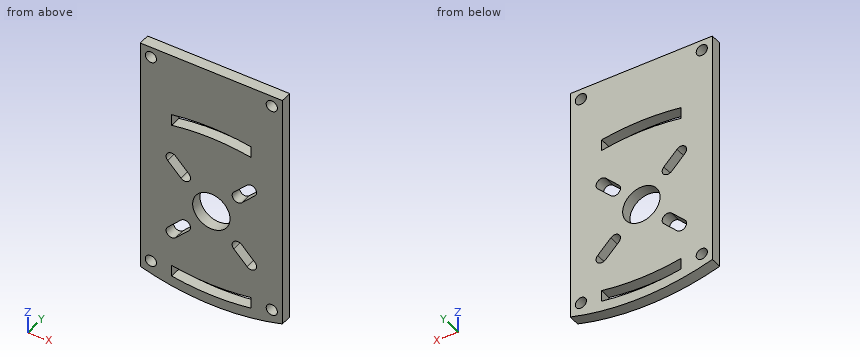
```python
from build123d import *

# Parameters (mm, degrees)
SKETCH_1_R      = 5
SKETCH_1_R_2    = 1.5
EXTRUDE_2_DEPTH = 3


with BuildPart() as part:
    # 草图1 → 凸台-拉伸2 (new body)
    with BuildSketch(Plane(origin=(0, 0, 0), x_dir=(1, 0, 0), z_dir=(0, 1, 0))):
        with BuildLine():
            Line((0, 0), (19, 0))
            Line((19, 0), (19, 64))
            ThreePointArc((19, 64), (0, 66.760766922), (-19, 64))
            Line((-19, 64), (-19, 0))
            Line((-19, 0), (0, 0))
        make_face()
        with Locations(Location((0, 40, 0), (0, 0, 270))):
            Circle(SKETCH_1_R, mode=Mode.SUBTRACT)
        with Locations(Location((-16.171572875, 2.828427125, 0), (0, 0, 270))):
            Circle(SKETCH_1_R_2, mode=Mode.SUBTRACT)
        with Locations(Location((-16.171572875, 61.171572875, 0), (0, 0, 270))):
            Circle(SKETCH_1_R_2, mode=Mode.SUBTRACT)
        with Locations(Location((16.171572875, 61.171572875, 0), (0, 0, 90))):
            Circle(SKETCH_1_R_2, mode=Mode.SUBTRACT)
        with Locations(Location((16.171572875, 2.828427125, 0), (0, 0, 90))):
            Circle(SKETCH_1_R_2, mode=Mode.SUBTRACT)
        with BuildLine():
            Line((10.606601718, 19.929208429), (10.606601718, 16.885025549))
            ThreePointArc((10.606601718, 16.885025549), (0, 16), (-10.606601718, 16.885025549))
            Line((-10.606601718, 16.885025549), (-10.606601718, 19.929208429))
            ThreePointArc((-10.606601718, 19.929208429), (0, 19), (10.606601718, 19.929208429))
        make_face(mode=Mode.SUBTRACT)
        with BuildLine():
            Line((-8.131727984, 46.01040764), (-11.66726189, 49.545941546))
            ThreePointArc((-11.66726189, 49.545941546), (-11.66726189, 51.66726189), (-9.545941546, 51.66726189))
            Line((-9.545941546, 51.66726189), (-6.01040764, 48.131727984))
            ThreePointArc((-6.01040764, 48.131727984), (-6.01040764, 46.01040764), (-8.131727984, 46.01040764))
        make_face(mode=Mode.SUBTRACT)
        with BuildLine():
            Line((6.01040764, 48.131727984), (9.545941546, 51.66726189))
            ThreePointArc((9.545941546, 51.66726189), (11.66726189, 51.66726189), (11.66726189, 49.545941546))
            Line((11.66726189, 49.545941546), (8.131727984, 46.01040764))
            ThreePointArc((8.131727984, 46.01040764), (6.01040764, 46.01040764), (6.01040764, 48.131727984))
        make_face(mode=Mode.SUBTRACT)
        with BuildLine():
            Line((8.131727984, 33.98959236), (11.66726189, 30.454058454))
            ThreePointArc((11.66726189, 30.454058454), (11.66726189, 28.33273811), (9.545941546, 28.33273811))
            Line((9.545941546, 28.33273811), (6.01040764, 31.868272016))
            ThreePointArc((6.01040764, 31.868272016), (6.01040764, 33.98959236), (8.131727984, 33.98959236))
        make_face(mode=Mode.SUBTRACT)
        with BuildLine():
            Line((-6.01040764, 31.868272016), (-9.545941546, 28.33273811))
            ThreePointArc((-9.545941546, 28.33273811), (-11.66726189, 28.33273811), (-11.66726189, 30.454058454))
            Line((-11.66726189, 30.454058454), (-8.131727984, 33.98959236))
            ThreePointArc((-8.131727984, 33.98959236), (-6.01040764, 33.98959236), (-6.01040764, 31.868272016))
        make_face(mode=Mode.SUBTRACT)
        with BuildLine():
            Line((-10.606601718, 60.070791571), (-10.606601718, 63.114974451))
            ThreePointArc((-10.606601718, 63.114974451), (0, 64), (10.606601718, 63.114974451))
            Line((10.606601718, 63.114974451), (10.606601718, 60.070791571))
            ThreePointArc((10.606601718, 60.070791571), (0, 61), (-10.606601718, 60.070791571))
        make_face(mode=Mode.SUBTRACT)
    extrude(amount=EXTRUDE_2_DEPTH)


solid = part.part
```
For this review, take the finished solid that the model builds, in its own axes (mm). Round coordinates to 2 decimals unless told otherwise and drop trailing zeros. Write each loop counter-clockwise with the first axis right and the second up, starting at its lowest first coordinate (ties: lowest second). Pieces come first, ordered by that corner, then holes. Notation, with made-up numbers: (89, 72.5) - (110, 72.5) arc R9 cw to (110, 89.5) - close; hole circle Ø6 at (46, 6.5). An arc over 180 degrees is marked (long way). Use CSV: the item, a comma, the result in double quotes.
1) Add section C-C on y = 1.1. Count the separate pieces of the cut face and the enclosed holes in it, and give its area (3 significant figures).
Conclusion:
separate pieces,"1"
enclosed holes,"11"
area,"2,180 mm^2"
2) Add section A-A on z = -40. Write out the cut boundary in (x, y), and give its area (3 significant figures).
Conclusion:
outline,"(-19, 0) - (-5, 0) - (-5, 3) - (-19, 3) - close; (5, 0) - (19, 0) - (19, 3) - (5, 3) - close"
area,"84.0 mm^2"
3) Clearance check with a flat-ended pin moving along its axis: pin 1 Ø2.5 at (x, z) = (-16.17, -61.17) entering from +Y. State where the tip first meets the part, or that it passes through.
Conclusion:
pin 1,"passes through"
4) Add section D-D on x = 4. Write out the cut boundary in (y, z), and give its area (3 significant figures).
Conclusion:
outline,"(0, -66.64) - (3, -66.64) - (3, -63.87) - (0, -63.87) - close; (0, -60.87) - (3, -60.87) - (3, -43) - (0, -43) - close; (0, -37) - (3, -37) - (3, -19.13) - (0, -19.13) - close; (0, -16.13) - (3, -16.13) - (3, 0) - (0, 0) - close"
area,"164 mm^2"
5) Add section B-B on x = 0. Write out the cut boundary in (y, z).
Conclusion:
outline,"(0, -66.76) - (3, -66.76) - (3, -64) - (0, -64) - close; (0, -61) - (3, -61) - (3, -45) - (0, -45) - close; (0, -35) - (3, -35) - (3, -19) - (0, -19) - close; (0, -16) - (3, -16) - (3, 0) - (0, 0) - close"
6) Wall thickness on line 1 along X through (y, z) = (0.2, -62.5); line 2 along X through (y, z) = (0.7, -61.5); line 3 along X through (y, z) = (2.65, -31): over which ranges is each line inside the solid? List them lowest first. Write a range as from..to.
Conclusion:
line 1,"x = -19..-16.87, -15.47..-10.61, 10.61..15.47, 16.87..19"
line 2,"x = -19..-17.64, -14.71..-10.61, 10.61..14.71, 17.64..19"
line 3,"x = -19..-11.12, -6.88..6.88, 11.12..19"
